Can you work these out from the model? Positions are in its coordinate system, mm. Face numbers are marked on the shaded views. A direction names the side the tool comes from. Give positions to 0.01 mm unless a question says otherwise; leave off trailing zeros. Loops run counter-clockwise (first coordinate to the right, second up) from the corner with the lowest first, then second, coordinate; pieces in that order, holes last. Notation, with made-up numbers: (1.25, 32.5) -> (52.25, 32.5) arc R13 ccw to (52.25, 39.5) -> close; hole circle Ø8 at (-13, 53). An arc over 180 degrees is marked (long way). Return JSON: item names as keys, results as strings. Group by question number.
Q1. Suppose I cut it at C-C, the plane x = 23. Please give me the cut outline in (y, z), and give its area (3 significant figures).
Q2. Suppose I cut it at D-D, the plane z = -25. Please give me the cut outline in (x, y).
Q3. Which directions (+Z, -Z, +X, -X, +Y, -Y) give clear straight access to the entire face, cutting with the end or side of a thin tool? Please do the marked faces 1, 2, 3 and 4.
Q4. I need wall thicknesses on line 1 along Z through (x, y) = (9, -45); line 2 along Y through (x, z) = (33, -26.75); line 3 along X through (y, z) = (6, -27.5). Which ranges of each line are inside material? Lowest first, please. Write a range as [from, to].
Q5. Suppose I cut it at B-B, the plane z = -20. Please give me the cut outline in (x, y).
Q6. Will these pins go through, and if not, where does the flat tip stop? pin 1 (7.5 mm diameter, centred on y = -50.5, z = -21, fed in from +X); pin 2 (3 mm diameter, centred on x = 14.5, z = -28, fed in from +Y); pin 3 (1 mm diameter, centred on y = -15, z = -12, fed in from +X).
Q7. Suppose I cut it at A-A, the plane y = 5. Please give me the cut outline in (x, z), and give its area (3 significant figures).
```python
from build123d import *

# Parameters (mm, degrees)
BOSS_EXTRUDE1_START = -10
BOSS_EXTRUDE1_DEPTH = 20
SKETCH2_R           = 2.5
CUT_EXTRUDE1_DEPTH  = 79.319856997
FILLET1_R           = 3


with BuildPart() as part:
    # Sketch1 → Boss-Extrude1 (new body)
    with BuildSketch(Plane.XY.offset(BOSS_EXTRUDE1_START)):
        with BuildLine():
            Line((40, -5), (8, -5))
            Line((8, -5), (8, 15))
            Line((8, 15), (10, 15))
            Line((10, 15), (10, -3))
            Line((10, -3), (40, -3))
            ThreePointArc((40, -3), (57, -20), (40, -37))
            Line((40, -37), (10, -37))
            Line((10, -37), (10, -55))
            Line((10, -55), (8, -55))
            Line((8, -55), (8, -35))
            Line((8, -35), (40, -35))
            ThreePointArc((40, -35), (55, -20), (40, -5))
        make_face()
    extrude(amount=-BOSS_EXTRUDE1_DEPTH)

    # Sketch2 → Cut-Extrude1 (cut, through all)
    with BuildSketch(Plane(origin=(10, 0, 0), x_dir=(0, 0, -1), z_dir=(1, 0, 0))):
        with Locations(Location((20, 5, 0), (0, 0, 90))):
            Circle(SKETCH2_R)
        with Locations(Location((20, -45, 0), (0, 0, 90))):
            Circle(SKETCH2_R)
    extrude(amount=-CUT_EXTRUDE1_DEPTH, mode=Mode.SUBTRACT)

    # Fillet1
    fillet1_edges = [part.edges().sort_by_distance(p)[0] for p in [
        (10, -37, -20),
        (8, -35, -20),
        (8, -5, -20),
        (10, -3, -20),
    ]]
    fillet(fillet1_edges, radius=FILLET1_R)


solid = part.part
```
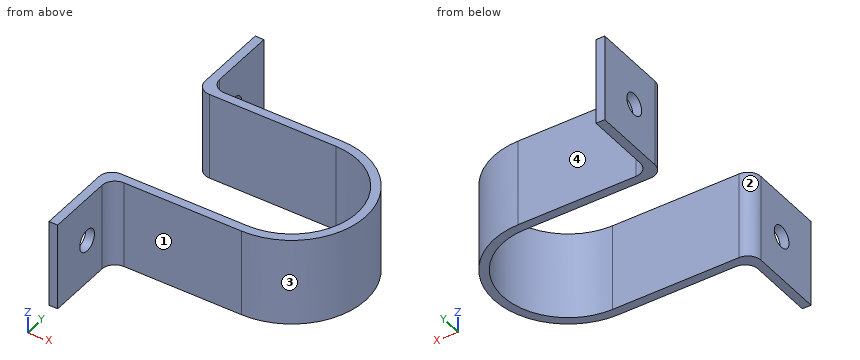
Ans:
{
 "1": {"outline": "(-37, -30) -> (-35, -30) -> (-35, -10) -> (-37, -10) -> close; (-5, -30) -> (-3, -30) -> (-3, -10) -> (-5, -10) -> close", "area": "80.0 mm^2"},
 "2": {"outline": "(8, -55) -> (10, -55) -> (10, -40) arc R3 cw to (13, -37) -> (40, -37) arc R17 ccw to (40, -3) -> (13, -3) arc R3 cw to (10, 0) -> (10, 15) -> (8, 15) -> (8, -2) arc R3 ccw to (11, -5) -> (40, -5) arc R15 cw to (40, -35) -> (11, -35) arc R3 ccw to (8, -38) -> close"},
 "3": {"face 1": "+Z, -Z, +X, -Y", "face 2": "+Z, -Z, -X", "face 3": "+Z, -Z, +X", "face 4": "+Z, -Z, +X, +Y"},
 "4": {"line 1": "z = [-30, -22.5], [-17.5, -10]", "line 2": "y = [-37, -35], [-5, -3]", "line 3": "x = [8, 10]"},
 "5": {"outline": "(8, -55) -> (10, -55) -> (10, -47.5) -> (8, -47.5) -> close; (8, -42.5) -> (10, -42.5) -> (10, -40) arc R3 cw to (13, -37) -> (40, -37) arc R17 ccw to (40, -3) -> (13, -3) arc R3 cw to (10, 0) -> (10, 2.5) -> (8, 2.5) -> (8, -2) arc R3 ccw to (11, -5) -> (40, -5) arc R15 cw to (40, -35) -> (11, -35) arc R3 ccw to (8, -38) -> close; (8, 7.5) -> (10, 7.5) -> (10, 15) -> (8, 15) -> close"},
 "6": {"pin 1": "stops at x = 10", "pin 2": "stops at y = -3", "pin 3": "stops at x = 56.39"},
 "7": {"outline": "(8, -30) -> (10, -30) -> (10, -22.5) -> (8, -22.5) -> close; (8, -17.5) -> (10, -17.5) -> (10, -10) -> (8, -10) -> close", "area": "30.0 mm^2"}
}
